from build123d import *

# Parameters (mm, degrees)
SKETCH_1_W               = 42
SKETCH_1_H               = 42
EXTRUDE_1_DEPTH          = 38
SKETCH_2_R               = 11
EXTRUDE_2_DEPTH          = 2
SKETCH_3_R               = 2.5
EXTRUDE_3_DEPTH          = 20
CUT_EXTRUDE_START        = -15
CUT_EXTRUDE_1_DEPTH      = 15
SKETCH_5_R               = 1.5
CUT_EXTRUDE_2_DEPTH      = 4.5
PATTERN_CIRCULAR_1_COUNT = 4
SKETCH_6_W               = 16
SKETCH_6_H               = 6
EXTRUDE_4_DEPTH          = 10
CHAMFER_1_SIZE           = 4


with BuildPart() as part:
    # 草图1 → 凸台-拉伸1 (new body)
    with BuildSketch(Plane(origin=(0, 0, 0), x_dir=(1, 0, 0), z_dir=(0, 1, 0))):
        Rectangle(SKETCH_1_W, SKETCH_1_H)
    extrude(amount=EXTRUDE_1_DEPTH)

    # 草图2 → 凸台-拉伸2 (add)
    with BuildSketch(Plane(origin=(0, 38, 0), x_dir=(1, 0, 0), z_dir=(0, 1, 0))):
        with Locations(Location((0, 0, 0), (0, 0, 270))):
            Circle(SKETCH_2_R)
    extrude(amount=EXTRUDE_2_DEPTH)

    # 草图3 → 凸台-拉伸3 (add)
    with BuildSketch(Plane(origin=(0, 40, 0), x_dir=(1, 0, 0), z_dir=(0, 1, 0))):
        with Locations(Location((0, 0, 0), (0, 0, 270))):
            Circle(SKETCH_3_R)
    extrude(amount=EXTRUDE_3_DEPTH)

    # 草图4 → 切除-拉伸1 (cut)
    with BuildSketch(Plane(origin=(0, 60, 0), x_dir=(1, 0, 0), z_dir=(0, 1, 0)).offset(CUT_EXTRUDE_START)):
        with BuildLine():
            Line((-1.5, 2), (1.5, 2))
            ThreePointArc((1.5, 2), (0, 2.5), (-1.5, 2))
        make_face()
    extrude(amount=CUT_EXTRUDE_1_DEPTH, mode=Mode.SUBTRACT)

    # 草图5 → 切除-拉伸2 (cut)
    with BuildSketch(Plane(origin=(0, 38, 0), x_dir=(1, 0, 0), z_dir=(0, 1, 0))):
        with Locations(Location((15.5, 15.5, 0), (0, 0, 270))):
            Circle(SKETCH_5_R)
    cut_extrude_2 = extrude(amount=-CUT_EXTRUDE_2_DEPTH, mode=Mode.SUBTRACT)

    # 阵列(圆周)1: 切除-拉伸2 ×4 about axis
    pattern_circular_1_axis = Axis((0, 0, 0), (0, 1, 0))
    for i in range(1, PATTERN_CIRCULAR_1_COUNT):
        add(cut_extrude_2.rotate(pattern_circular_1_axis, i * 360 / PATTERN_CIRCULAR_1_COUNT), mode=Mode.SUBTRACT)

    # 草图6 → 凸台-拉伸4 (add)
    with BuildSketch(Plane.XZ):
        with Locations((0, 24)):
            Rectangle(SKETCH_6_W, SKETCH_6_H)
    extrude(amount=-EXTRUDE_4_DEPTH)

    # 倒角1
    chamfer_1_edges = [part.edges().sort_by_distance(p)[0] for p in [
        (21, 19, 21),
        (-21, 19, 21),
        (-21, 19, -21),
        (21, 19, -21),
    ]]
    chamfer(chamfer_1_edges, length=CHAMFER_1_SIZE)


solid = part.part
Design review of the part built by this model. Coordinates are the model's own, in mm. A direction names the side the tool comes from. Give positions to 0.01 mm unless a question says otherwise; leave off trailing zeros. Order: outer loops, then holes, each group sorted by start corner. A loop starts at its lowest first (then second) coordinate and runs counter-clockwise, first axis right, second up. Notation, with made-up numbers: (20.25, 85.5) - (41.25, 85.5) arc R22 cw to (41.25, 95.5) - close; hole circle Ø10 at (11.5, 89). An arc over 180 degrees is marked (long way). Write item = value, one per line. Start each with the question number.
Q1. We need section D-D on x = 15.5. State the section outline as (y, z) points, plus the area to 3 significant figures.
Q2. We need section C-C on y = 28.5. State the section outline as (x, z) points, plus the area to 3 significant figures.
Q3. To check wall thickness, follow L1, parallel to X at y = 35.6, z = -15.5; L2, parallel to Z at x = 15, y = 36. State the ranges of each line that lie inside material, in increasing order. Write a range as from..to.
Q4. Tool access review of faces 1 (the face through (0, 52, -2)), 2 (the face through (0.751, 49.86, 2.385)), 3 (the face through (8, 5, 24)): name each direction out of +Z, -Z, +X, -X, +Y, -Y from which nothing blocks a thin tool from reaching the whole face with its end or side.
Q5. We need section B-B on z = 15.5. State the section outline as (x, y) points.
Q6. We need section A-A on x = 0. State the section outline as (y, z) points, plus the area to 3 significant figures.
Q7. Mouldability with a two-part tool opening along X and no side actions: class faces 4 (the face through (-17, 35.78, -15.57)), 5 (the face through (-10, 38, -10)), 6 (the face through (19, 19, -19)) as released by +X, released by -X, zero draft, split by the parting line, or undercut.
Q8. Clearance check with flat-ended pins moving along their axes: pin 1 Ø2.5 at (x, z) = (-15.5, 15.5) entering from +Y; pin 2 Ø2.5 at (x, z) = (-15.5, -15) entering from +Y; pin 3 Ø2 at (y, z) = (15, 21.5) entering from +X; pin 4 Ø11 at (x, z) = (4, -5.5) entering from +Y. State where each tip first meets the part, or that it passes through.
Working result:
q1.outline = (0, -21) - (38, -21) - (38, -17) - (33.5, -17) - (33.5, -14) - (38, -14) - (38, 14) - (33.5, 14) - (33.5, 17) - (38, 17) - (38, 21) - (0, 21) - close
q1.area = 1,570 mm²
q2.outline = (-21, -17) - (-17, -21) - (17, -21) - (21, -17) - (21, 17) - (17, 21) - (-17, 21) - (-21, 17) - close
q2.area = 1,730 mm²
q3.L1 = -21..-17, -14..14, 17..21
q3.L2 = -21..-16.91, -14.09..14.09, 16.91..21
q4.face_1 = -Z, +X, -X, +Y
q4.face_2 = +Y
q4.face_3 = +Z, +X, +Y, -Y
q5.outline = (-21, 0) - (21, 0) - (21, 38) - (17, 38) - (17, 33.5) - (14, 33.5) - (14, 38) - (-14, 38) - (-14, 33.5) - (-17, 33.5) - (-17, 38) - (-21, 38) - close
q6.outline = (0, -21) - (38, -21) - (38, -11) - (40, -11) - (40, -2.5) - (45, -2.5) - (45, -2) - (60, -2) - (60, 2.5) - (40, 2.5) - (40, 11) - (38, 11) - (38, 21) - (10, 21) - (10, 27) - (0, 27) - close
q6.area = 1,790 mm²
q7.face_4 = undercut
q7.face_5 = zero draft
q7.face_6 = released by +X
q8.pin_1 = 33.5
q8.pin_2 = 38
q8.pin_3 = 17.5
q8.pin_4 = 60
